Model file for the job. Use its own axes, mm. A direction names the side the tool comes from. Round coordinates to 2 decimals unless told otherwise and drop trailing zeros. Order: outer loops, then holes, each group sorted by start corner. A loop starts at its lowest first (then second) coordinate and runs counter-clockwise, first axis right, second up. Notation, with made-up numbers: (73, -16.5) - (112, -16.5) arc R23 cw to (112, -2.5) - close; hole circle Ø6 at (67, 65.25). An arc over 180 degrees is marked (long way). Put each result on its own line as item: value. Start each with the question number.
Item 1: Saw through at D-D on x = -20. List the corners of the cut face in (y, z), plus the area to 3 significant figures.
Item 2: Saw through at C-C on y = -26.5. List the corners of the cut face in (x, z).
Item 3: Saw through at B-B on z = 11. List the corners of the cut face in (x, y).
Item 4: Probe probe 1 along Y at (x, z) = (48, 3.2); probe 2 along Y at (x, z) = (-48, 1.9); probe 3 along Z at (x, y) = (6, -12.5). List the from-to ranges inside material, lowest first.
Item 5: Saw through at A-A on x = -48. List the corners of the cut face in (y, z), plus the area to 4 significant figures.
Item 6: Pin check, flat tips, straight feed: pin 1 Ø1.9 at (y, z) = (-14, 10.5) entering from +X; pin 2 Ø1 at (y, z) = (-21.5, 7) entering from +X; pin 3 Ø3 at (y, z) = (-11.5, 10.5) entering from -X. Stop position of each tip, or through.
Item 7: Mould opens along Y. For faces 3 (the face through (53, -2, 3)), 4 (the face through (-49.5, -30.93, 2.22)), 5 (the face through (-52, -35, 2)), 6 (the face through (0, -18, 5)) say: pulls with the +Y half, pulls with the -Y half, needs draft (parallel to the pull), parting line crosses it, or undercut.
Item 8: Which spindle directions (+Z, -Z, +X, -X, +Y, -Y) get a long thin tool onto all of the face, cutting with end or side? Do faces 1 (the face through (-12, -18, 12)), 2 (the face through (39, -18, 5)). Say none if no direction does.
```python
from build123d import *

# Parameters (mm, degrees)
F1_DEPTH = 36
F2_SIZE  = 5
F3_R     = 1.5
F4_DEPTH = 13.1
F5_SIZE  = 0.5
F6_R     = 5


with BuildPart() as f1:
    # F0 (on Front) → F1 (new body)
    with BuildSketch(Plane.XZ):
        Polygon((-54, 0), (0, 0), (54, 0), (54, 5), (24, 5), (24, 12), (5, 12), (5, 8.2), (9.5, 8.2), (9.5, 5), (0, 5), (-9.5, 5), (-9.5, 8.2), (-5, 8.2), (-5, 12), (-24, 12), (-24, 5), (-54, 5), align=None)
    extrude(amount=F1_DEPTH)

    # F2
    f2_edges = [f1.edges().sort_by_distance(p)[0] for p in [
        (24, -18, 12),
        (-24, -18, 12),
    ]]
    chamfer(f2_edges, length=F2_SIZE)

    # F3 (on Top) → F4 (cut)
    with BuildSketch(Plane.XY):
        with Locations((-48, -5)):
            Circle(F3_R)
        with Locations((-48, -31)):
            Circle(F3_R)
        with Locations((48, -5)):
            Circle(F3_R)
        with Locations((48, -30)):
            Circle(F3_R)
    extrude(amount=F4_DEPTH, mode=Mode.SUBTRACT)

    # F5
    f5_edges = [f1.edges().sort_by_distance(p)[0] for p in [
        (-49.5, -5, 5),
        (-49.5, -31, 5),
        (46.5, -5, 5),
        (46.5, -30, 5),
    ]]
    chamfer(f5_edges, length=F5_SIZE)

    # F6
    f6_edges = [f1.edges().sort_by_distance(p)[0] for p in [
        (-54, 0, 2.5),
        (-54, -36, 2.5),
        (54, -36, 2.5),
        (54, 0, 2.5),
    ]]
    fillet(f6_edges, radius=F6_R)


solid = f1.part
```
Results found:
1. outline: (-36, 0) - (0, 0) - (0, 11) - (-36, 11) - close
1. area: 396 mm²
2. outline: (-54, 0) - (54, 0) - (54, 5) - (24, 5) - (24, 7) - (19, 12) - (5, 12) - (5, 8.2) - (9.5, 8.2) - (9.5, 5) - (-9.5, 5) - (-9.5, 8.2) - (-5, 8.2) - (-5, 12) - (-19, 12) - (-24, 7) - (-24, 5) - (-54, 5) - close
3. outline: (-20, -36) - (-5, -36) - (-5, 0) - (-20, 0) - close; (5, -36) - (20, -36) - (20, 0) - (5, 0) - close
4. probe 1: y = -36 to -31.5, -28.5 to -6.5, -3.5 to 0
4. probe 2: y = -36 to -32.5, -29.5 to -6.5, -3.5 to 0
4. probe 3: z = 0 to 5, 8.2 to 12
5. outline: (-36, 0) - (-32.5, 0) - (-32.5, 4.5) - (-33, 5) - (-36, 5) - close; (-29.5, 0) - (-6.5, 0) - (-6.5, 4.5) - (-7, 5) - (-29, 5) - (-29.5, 4.5) - close; (-3.5, 0) - (0, 0) - (0, 5) - (-3, 5) - (-3.5, 4.5) - close
5. area: 149.5 mm²
6. pin 1: stops at x = 21.45
6. pin 2: stops at x = 24
6. pin 3: stops at x = -22
7. face 3: pulls with the +Y half
7. face 4: undercut
7. face 5: pulls with the -Y half
7. face 6: needs draft
8. face 1: +Z, +X, -X, +Y, -Y
8. face 2: +Z, +X, +Y, -Y
